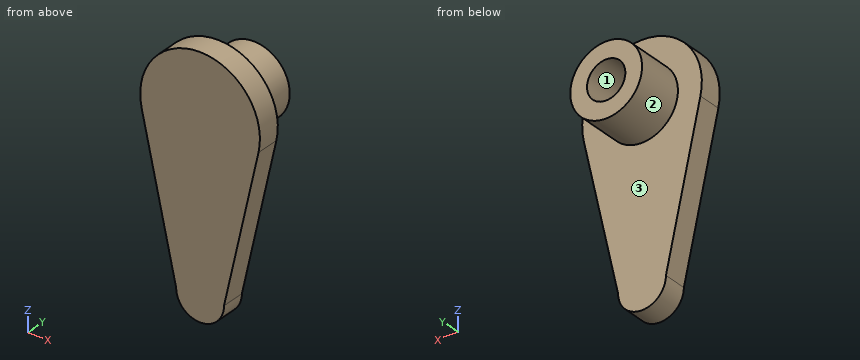
Autodesk Inventor part; units mm, degrees
ref_plane "YZ Plane" through (0, 0, 0) normal (1, 0, 0) x (0, 1, 0)
ref_plane "XZ Plane" through (0, 0, 0) normal (0, 1, 0) x (-1, 0, 0)
ref_plane "XY Plane" through (0, 0, 0) normal (0, 0, 1) x (1, 0, 0)
sketch "Sketch1" plane through (0, 0, 0) normal (0, 1, 0) x (-1, 0, 0)
  point P0 (0, 0)
sketch "Sketch2" plane through (0, 0, 0) normal (0, 1, 0) x (-1, 0, 0)
  arc A0 (12.2002, -2.7214) -> (-12.2002, -2.7214) centre (0, 0) ccw
  arc A1 (-5, -35) -> (5, -35) centre (0, -35) ccw
  line L0 (5, -35) -> (12.2002, -2.7214)
  line L1 (-5, -35) -> (-12.2002, -2.7214)
  line L2 (0, 0) -> (0, -12.5)
  line L3 (0, -30) -> (0, -35)
  dimension "d0" = 25
  dimension "d1" = 35
  dimension "d2" = 10
extrude "Extrusion1" add sketch "Sketch2" along normal blind 5
sketch "Sketch3" plane through (0, 5, 0) normal (0, 1, 0) x (1, 0, 0)
  circle A0 centre (0, 0) radius 4
  circle A1 centre (0, 0) radius 7.5
  dimension "d5" = 8
  dimension "d6" = 15
extrude "Extrusion2" add sketch "Sketch3" along normal blind 10
properties part number "connector1"
Can you work these out from the model? Positions are in its coordinate system, mm. Face numbers are marked on the shaded views. Coordinates: 2 decimals unless noted, no trailing zeros. Write each loop counter-clockwise with the first axis right and the second up, starting at its lowest first coordinate (ties: lowest second). Pieces come first, ordered by that corner, then holes. Notation, with made-up numbers: (26.25, 24) -> (50.25, 24) arc R17 ccw to (50.25, 36) -> close; hole circle Ø1 at (6.5, 45.25). An arc over 180 degrees is marked (long way). Answer as CSV lines item,"result".
1) If I drill on line 1 (Z direction, x = 0, y = 9.5); line 2 (X direction, y = 1, z = -38), over which ranges is the centre line in solid material (lowest first)? Write a range as from..to.
Check result:
line 1,"-7.5..-4, 4..7.5"
line 2,"-4..4"
2) If we mould it in two halves opening along X, with no side actions, what happens to the marked faces 1, 2 and 3? For each: +X half, -X half, draft (parallel to the pull), parting line (faces both ways), or undercut.
Check result:
face 1,"undercut"
face 2,"parting line"
face 3,"draft"
3) If we section it at B-B on y = 11: Please give me the cut outline in (x, z), then the cut area to 3 significant figures.
Check result:
outline,"circle Ø15 at (0, 0); hole circle Ø8 at (0, 0)"
area,"126 mm²"
4) If we section it at A-A on z = 0: Please give me the cut outline in (x, y).
Check result:
outline,"(-12.5, 0) -> (12.5, 0) -> (12.5, 5) -> (7.5, 5) -> (7.5, 15) -> (4, 15) -> (4, 5) -> (-4, 5) -> (-4, 15) -> (-7.5, 15) -> (-7.5, 5) -> (-12.5, 5) -> close"
5) If we section it at D-D on y = 1.75: Please give me the cut outline in (x, z).
Check result:
outline,"(-12.2, -2.72) -> (-5, -35) arc R5 ccw to (5, -35) -> (12.2, -2.72) arc R12.5 ccw (long way) to start"
6) Will this pin go through, and if not, where does the flat tip stop? P1, Ø5, axis at y = 6, z = -13.5, coming from the +X side.
Check result:
P1,"x = 10.31"
7) If we section it at C-C on x = -1.5: Please give me the cut outline in (y, z), then the cut area to 3 significant figures.
Check result:
outline,"(0, -39.77) -> (5, -39.77) -> (5, -7.35) -> (15, -7.35) -> (15, -3.71) -> (5, -3.71) -> (5, 3.71) -> (15, 3.71) -> (15, 7.35) -> (5, 7.35) -> (5, 12.41) -> (0, 12.41) -> close"
area,"334 mm²"
